Design review of the part built by this model. Coordinates are the model's own, in mm. Give positions to 0.01 mm unless a question says otherwise; leave off trailing zeros. Loops run counter-clockwise (first coordinate to the right, second up) from the corner with the lowest first, then second, coordinate; pieces in that order, holes last. Notation, with made-up numbers: M 49.5,43 L 87.5,43 A30 ccw 87.5,65 Z; hole C 70.5,68 d10. An arc over 180 degrees is marked long. Use a Markdown table: item, result. Add a question column.
(1) Insertion check: pin 1 Ø13.5 at (y, z) = (0, 138) entering from +X; pin 2 Ø5 at (x, y) = (-13.5, -2.5) entering from -Z. Each pin has a flat end and moves straight along its axis. Give the tip position at first contact, or say it passes through.
(2) Add section C-C, the plane x = -7.5. Give the boundary of the cut face in (y, z).
(3) Add section A-A, the plane z = -20. Give the boundary of the cut face in (x, y), then the cut area to 3 significant figures.
(4) Add section B-B, the plane y = 0. Give the boundary of the cut face in (x, z), then the cut area to 3 significant figures.
(5) For probe 1 along Y at (x, z) = (-11.5, -32); probe 2 along Z at (x, y) = (-7.5, -9.5); probe 3 along Z at (x, y) = (-10.25, 0), list the stretches that pass through material, from the lowest coordinate up.
```python
from build123d import *

# Parameters (mm, degrees)
F0_R          = 5.25
F1_DEPTH      = 15
F2_R          = 3
F3_DEPTH      = 25
F3_DEPTH_BACK = 25


with BuildPart() as f1:
    # F0 (on Right) → F1 (new body)
    with BuildSketch(Plane.YZ):
        Polygon((-6, -40), (-6, 0), (6, 0), (6, -40), (16, -40), (16, 150), (-16, 150), (-16, -40), align=None)
        with Locations((0, 138)):
            Circle(F0_R, mode=Mode.SUBTRACT)
    extrude(amount=-F1_DEPTH)

    # F2 (on Front) → F3 (cut, two sides)
    with BuildSketch(Plane.XZ) as f3_sk:
        with Locations((-7.5, -20)):
            Circle(F2_R)
    extrude(amount=-F3_DEPTH, mode=Mode.SUBTRACT)
    extrude(f3_sk.sketch, amount=F3_DEPTH_BACK, mode=Mode.SUBTRACT)


solid = f1.part
```
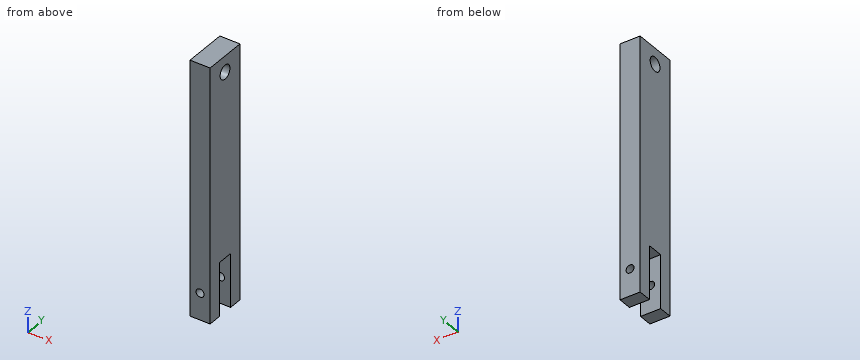
Established:
| question | item | result |
|---|---|---|
| 1 | pin 1 | x = 0 |
| 1 | pin 2 | z = 0 |
| 2 | outline | M -16,-40 L -6,-40 L -6,-23 L -16,-23 Z; M -16,-17 L -6,-17 L -6,0 L 6,0 L 6,-17 L 16,-17 L 16,150 L -16,150 Z; M 6,-40 L 16,-40 L 16,-23 L 6,-23 Z; hole C 0,138 d10.5 |
| 3 | outline | M -15,-16 L -10.5,-16 L -10.5,-6 L -15,-6 Z; M -15,6 L -10.5,6 L -10.5,16 L -15,16 Z; M -4.5,-16 L 0,-16 L 0,-6 L -4.5,-6 Z; M -4.5,6 L 0,6 L 0,16 L -4.5,16 Z |
| 3 | area | 180 mm^2 |
| 4 | outline | M -15,0 L 0,0 L 0,132.75 L -15,132.75 Z; M -15,143.25 L 0,143.25 L 0,150 L -15,150 Z |
| 4 | area | 2,090 mm^2 |
| 5 | probe 1 | -16 to -6, 6 to 16 |
| 5 | probe 2 | -40 to -23, -17 to 150 |
| 5 | probe 3 | 0 to 132.75, 143.25 to 150 |
